```python
from build123d import *

# Parameters (mm, degrees)
SKETCH1_W                           = 23
SKETCH1_H                           = 15
BOSS_EXTRUDE1_DEPTH                 = 3
BOSS_EXTRUDE2_DEPTH                 = 12.5
BOSS_EXTRUDE2_DEPTH_BACK            = 3
SKETCH2_W                           = 3
SKETCH2_H                           = 15
BOSS_EXTRUDE3_DEPTH                 = 10
TAP_START                           = -2.5
TAP_DRILL_FOR_M2X0_4_TAP1_OUTLINE_R = 0.8
TAP_DRILL_FOR_M2X0_4_TAP1_DEPTH     = 10
SKETCH6_W                           = 29
SKETCH6_H                           = 20
BOSS_EXTRUDE4_DEPTH                 = 3
SKETCH7_W                           = 10
SKETCH7_H                           = 10
CUT_EXTRUDE1_DEPTH                  = 35.301056835
CUT_EXTRUDE2_DEPTH                  = 2
F_4_0_4_DIAMETER_HOLE1_D            = 4
F_4_0_4_DIAMETER_HOLE1_DEPTH        = 10
F_4_0_4_DIAMETER_HOLE1_TIP          = 1.201721238
SKETCH12_W                          = 29
SKETCH12_H                          = 15
BOSS_EXTRUDE5_DEPTH                 = 2
SKETCH13_W                          = 3
SKETCH13_H                          = 7
CUT_EXTRUDE4_DEPTH                  = 3.5


# Read off the part's stored shape, not the designer's step: Tap Drill for M2x0.4 Tap1
with BuildPart() as part:
    # Sketch1 → Boss-Extrude1 (new body)
    with BuildSketch(Plane(origin=(0, 0, 0), x_dir=(1, 0, 0), z_dir=(0, 1, 0))):
        Rectangle(SKETCH1_W, SKETCH1_H)
    extrude(amount=BOSS_EXTRUDE1_DEPTH)

    # Sketch2 → Boss-Extrude2 (add, two sides: drawn at the far end of the back side and taken through both)
    with BuildSketch(Plane(origin=(0, 3, 0), x_dir=(1, 0, 0), z_dir=(0, 1, 0)).offset(-BOSS_EXTRUDE2_DEPTH_BACK)):
        with Locations((13, 0)):
            Rectangle(SKETCH2_W, SKETCH2_H)
        with Locations((-13, 0)):
            Rectangle(SKETCH2_W, SKETCH2_H)
    extrude(amount=BOSS_EXTRUDE2_DEPTH + BOSS_EXTRUDE2_DEPTH_BACK)

    # Sketch3 → Boss-Extrude3 (add)
    with BuildSketch(Plane.XY.offset(7.5)):
        with BuildLine():
            ThreePointArc((16.25, 9.5), (15.765564437, 10.979019946), (14.5, 11.884848004))
            Line((14.5, 11.884848004), (14.5, 7.115151996))
            ThreePointArc((14.5, 7.115151996), (15.765564437, 8.020980054), (16.25, 9.5))
        make_face()
        with BuildLine():
            Line((-14.5, 7.115151996), (-14.5, 11.884848004))
            ThreePointArc((-14.5, 11.884848004), (-16.25, 9.5), (-14.5, 7.115151996))
        make_face()
    extrude(amount=-BOSS_EXTRUDE3_DEPTH)

    # Tap Drill for M2x0.4 Tap1 outline → Tap Drill for M2x0.4 Tap1 (cut)
    with BuildSketch(Plane.XY.offset(TAP_START)):
        with Locations((-13.75, 9.5)):
            Circle(TAP_DRILL_FOR_M2X0_4_TAP1_OUTLINE_R)
    extrude(amount=TAP_DRILL_FOR_M2X0_4_TAP1_DEPTH, mode=Mode.SUBTRACT)

    # Tap Drill for M2x0.4 Tap1 2 outline → Tap Drill for M2x0.4 Tap1 2 (revolve, cut)
    with BuildSketch(Plane(origin=(13.75, 9.5, 0), x_dir=(1, 0, 0), z_dir=(0, -1, 0))):
        Polygon((0, 7.5), (0, -2.980688495), (0.800001695, -2.499998981), (0.8, 7.5), align=None)
    revolve(axis=Axis((13.75, 9.5, 0), (0, 0, 1)), mode=Mode.SUBTRACT)

    # Sketch6 → Boss-Extrude4 (add)
    with BuildSketch(Plane.XZ):
        with Locations((0, 17.5)):
            Rectangle(SKETCH6_W, SKETCH6_H)
    extrude(amount=-BOSS_EXTRUDE4_DEPTH)

    # Sketch7 → Cut-Extrude1 (cut, through all)
    with BuildSketch(Plane(origin=(0, 3, 0), x_dir=(1, 0, 0), z_dir=(0, 1, 0))):
        with Locations((9.5, -22.5)):
            Rectangle(SKETCH7_W, SKETCH7_H)
    extrude(amount=-CUT_EXTRUDE1_DEPTH, mode=Mode.SUBTRACT)

    # Sketch8 → Cut-Extrude2 (cut)
    with BuildSketch(Plane.XZ.offset(-3)):
        Polygon((-5.767949192, 17), (-4.035898385, 20), (-5.767949192, 23), (-9.232050808, 23), (-10.964101615, 20), (-9.232050808, 17), align=None)
    extrude(amount=CUT_EXTRUDE2_DEPTH, mode=Mode.SUBTRACT)

    # Ø4.0 (4) Diameter Hole1
    with Locations(Plane(origin=(0, 0, 0), x_dir=(-1, 0, 0), z_dir=(0, -1, 0))):
        with Locations((7.5, -20)):
            Hole(F_4_0_4_DIAMETER_HOLE1_D / 2, depth=F_4_0_4_DIAMETER_HOLE1_DEPTH)
            with Locations((0, 0, -(F_4_0_4_DIAMETER_HOLE1_DEPTH + F_4_0_4_DIAMETER_HOLE1_TIP / 2))):  # 118° drill point
                Cone(0, F_4_0_4_DIAMETER_HOLE1_D / 2, F_4_0_4_DIAMETER_HOLE1_TIP, mode=Mode.SUBTRACT)

    # Sketch12 → Boss-Extrude5 (add)
    with BuildSketch(Plane(origin=(0, 15.5, 0), x_dir=(1, 0, 0), z_dir=(0, 1, 0))):
        Rectangle(SKETCH12_W, SKETCH12_H)
    extrude(amount=BOSS_EXTRUDE5_DEPTH)

    # Sketch13 → Cut-Extrude4 (cut)
    with BuildSketch(Plane(origin=(0, 0, -7.5), x_dir=(-1, 0, 0), z_dir=(0, 0, -1))):
        with Locations((-13, 9.25)):
            Rectangle(SKETCH13_W, SKETCH13_H)
    extrude(amount=-CUT_EXTRUDE4_DEPTH, mode=Mode.SUBTRACT)


solid = part.part
```
The model under review builds one solid part; all positions refer to its coordinate system, in mm. A direction names the side the tool comes from. Round coordinates to 2 decimals unless told otherwise and drop trailing zeros. Order: outer loops, then holes, each group sorted by start corner. A loop starts at its lowest first (then second) coordinate and runs counter-clockwise, first axis right, second up. Notation, with made-up numbers: (4.5, -8) -> (43.5, -8) arc R16 cw to (43.5, 11) -> close; hole circle Ø11 at (-19, -28). An arc over 180 degrees is marked (long way). One line per item, written item: value. Start each with the question number.
Q1. Clearance check with flat-ended pins moving along their axes: pin 1 Ø0.9 at (x, y) = (12.5, 10.5) entering from -Z; pin 2 Ø6.5 at (x, z) = (-7.5, 20) entering from +Y; pin 3 Ø0.8 at (x, y) = (-14, 9.5) entering from +Z. State where each tip first meets the part, or that it passes through.
Q2. Machinability: for faces 1 (the face through (15, 10, -2.5)), 2 (the face through (14.12, 8.79, 2.57)), 3 (the face through (13, 12.75, -6)), 4 (the face through (9, 2, 17.5)), which of the approach directions +Z, -Z, +X, -X, +Y, -Y give a long, thin tool a straight path to every point of the face, cutting with its end or side? Answer none if there is none.
Q3. Take a section at B-B (y = 8). Write out the cut boundary in (x, z).
Q4. Take a section at A-A (x = 1.5). Write out the cut boundary in (y, z), and give its area (3 significant figures).
Q5. Wall thickness on line 1 (Z direction, x = -7.5, y = 0.35); line 2 (Y direction, x = -13.75, z = 1); line 3 (X direction, y = 9.25, z = 3): over which ranges is each line inside the solid? List them lowest first.
Q6. Take a section at D-D (x = -7.5). Write out the cut boundary in (y, z), and give its area (3 significant figures).
Q7. Mouldability with a two-part tool opening along Z and no side actions: class faces 5 (the face through (-15, 10, -2.5)), 6 (the face through (11.5, 9, 0)), 7 (the face through (0, 16, 7.5)), 8 (the face through (-6.78, 1, 22.04)) as released by +Z, released by -Z, zero draft, split by the parting line, or undercut.
Q8. Take a section at C-C (z = 5.5). Write out the cut boundary in (x, y), and give its area (3 significant figures).
Reported:
1. pin 1: stops at z = -4
1. pin 2: stops at y = 3
1. pin 3: stops at z = -2.5
2. face 1: -Z, +X, +Y, -Y
2. face 2: +Z
2. face 3: -Z, +X
2. face 4: +Z, +X, +Y, -Y
3. outline: (-15.75, -2.5) -> (-14.5, -2.5) -> (-14.5, -7.5) -> (-11.5, -7.5) -> (-11.5, 7.5) -> (-15.75, 7.5) -> close; (11.5, -4) -> (14.5, -4) -> (14.5, -2.5) -> (15.75, -2.5) -> (15.75, 7.5) -> (11.5, 7.5) -> close
4. outline: (0, -7.5) -> (3, -7.5) -> (3, 27.5) -> (0, 27.5) -> close; (15.5, -7.5) -> (17.5, -7.5) -> (17.5, 7.5) -> (15.5, 7.5) -> close
4. area: 135 mm2
5. line 1: z = -7.5 to 18, 22 to 27.5
5. line 2: y = 0 to 8.7, 10.3 to 17.5
5. line 3: x = -16.24 to -14.51, -12.99 to -11.5, 11.5 to 12.99, 14.51 to 16.24
6. outline: (0, -7.5) -> (3, -7.5) -> (3, 17) -> (1, 17) -> (1, 18) -> (0, 18) -> close; (0, 22) -> (1, 22) -> (1, 23) -> (3, 23) -> (3, 27.5) -> (0, 27.5) -> close; (15.5, -7.5) -> (17.5, -7.5) -> (17.5, 7.5) -> (15.5, 7.5) -> close
6. area: 119 mm2
7. face 5: released by -Z
7. face 6: zero draft
7. face 7: released by +Z
7. face 8: undercut
8. outline: (-14.5, 0) -> (14.5, 0) -> (14.5, 7.12) arc R2.5 ccw to (14.5, 11.88) -> (14.5, 17.5) -> (-14.5, 17.5) -> (-14.5, 11.88) arc R2.5 ccw to (-14.5, 7.12) -> close; hole circle Ø1.6 at (-13.75, 9.5); hole (-11.5, 3) -> (11.5, 3) -> (11.5, 15.5) -> (-11.5, 15.5) -> close; hole circle Ø1.6 at (13.75, 9.5)
8. area: 228 mm2
